from build123d import *

# Parameters (mm, degrees)
F0_W     = 3.81
F0_H     = 88.9
F1_DEPTH = 7.62


with BuildPart() as f1:
    # F0 (on Top) → F1 (new body)
    with BuildSketch(Plane.XY):
        Polygon((12.7, 0), (0, 0), (0, -21.2725), (7.62, -21.2725), (7.62, -33.9725), (0, -33.9725), (0, -46.6725), (7.62, -46.6725), (7.62, -59.3725), (0, -59.3725), (0, -72.0725), (7.62, -72.0725), (7.62, -84.7725), (0, -84.7725), (0, -97.4725), (7.62, -97.4725), (7.62, -110.1725), (0, -110.1725), (0, -131.445), (12.7, -131.445), (12.7, -123.825), (25.4, -123.825), (25.4, -131.445), (38.1, -131.445), (38.1, -123.825), (50.8, -123.825), (50.8, -131.445), (63.5, -131.445), (63.5, -123.825), (76.2, -123.825), (76.2, -131.445), (88.9, -131.445), (88.9, -110.1725), (81.28, -110.1725), (81.28, -97.4725), (88.9, -97.4725), (88.9, -84.7725), (81.28, -84.7725), (81.28, -72.0725), (88.9, -72.0725), (88.9, -59.3725), (81.28, -59.3725), (81.28, -46.6725), (88.9, -46.6725), (88.9, -33.9725), (81.28, -33.9725), (81.28, -21.2725), (88.9, -21.2725), (88.9, 0), (76.2, 0), (76.2, -7.62), (63.5, -7.62), (63.5, 0), (50.8, 0), (50.8, -7.62), (38.1, -7.62), (38.1, 0), (25.4, 0), (25.4, -7.62), (12.7, -7.62), align=None)
        with Locations((17.145, -66.04)):
            Rectangle(F0_W, F0_H, mode=Mode.SUBTRACT)
        with Locations((24.003, -66.04)):
            Rectangle(F0_W, F0_H, mode=Mode.SUBTRACT)
        with Locations((30.861, -66.04)):
            Rectangle(F0_W, F0_H, mode=Mode.SUBTRACT)
        with Locations((37.719, -66.04)):
            Rectangle(F0_W, F0_H, mode=Mode.SUBTRACT)
        with Locations((51.181, -66.04)):
            Rectangle(F0_W, F0_H, mode=Mode.SUBTRACT)
        with Locations((58.039, -66.04)):
            Rectangle(F0_W, F0_H, mode=Mode.SUBTRACT)
        with Locations((64.897, -66.04)):
            Rectangle(F0_W, F0_H, mode=Mode.SUBTRACT)
        with Locations((71.755, -66.04)):
            Rectangle(F0_W, F0_H, mode=Mode.SUBTRACT)
    extrude(amount=F1_DEPTH)


solid = f1.part
The listing builds one solid part. Answer for the finished solid, in the listing's coordinates (mm). A direction names the side the tool comes from. Give positions to 0.01 mm unless a question says otherwise; leave off trailing zeros. Answer as a JSON object with one key per item and string values.
1. Find the intervals of material crossed by L1, parallel to Y at x = 84.5, z = 0.5 (1 decimal); L2, parallel to X at y = -7, z = 1.5; L3, parallel to Y at x = 57, z = 2.75 (3 decimals), in increasing order. Write a range as [from, to].
Determined:
{"L1": "[-131.4, -110.2], [-97.5, -84.8], [-72.1, -59.4], [-46.7, -34], [-21.3, 0]", "L2": "[0, 12.7], [25.4, 38.1], [50.8, 63.5], [76.2, 88.9]", "L3": "[-131.445, -110.49], [-21.59, 0]"}
2. For faces 4 (the flat face through (0, -40, 4)), 5 (the flat face through (4, -33.972, 4)), 6 (the flat face through (50.8, -4, 4)), 7 (the flat face through (70, -123.825, 4)), 8 (the flat face through (51, -110.49, 4)), determine the directions among +Z, -Z, +X, -X, +Y, -Y from which every point of the face is accessible in a straight line to the end or side of a thin tool.
Determined:
{"face 4": "+Z, -Z, -X, +Y, -Y", "face 5": "+Z, -Z, -X", "face 6": "+Z, -Z, +Y", "face 7": "+Z, -Z, -Y", "face 8": "+Z, -Z"}
3. Flat-ended cylindrical pins translate along their axes: pin 1 Ø1 at (y, z) = (-83, 4) entering from -X; pin 2 Ø2 at (y, z) = (-53.5, 2.5) entering from +X; pin 3 Ø4 at (x, z) = (72, 3.5) entering from +Y. Find the tip coordinate at first contact, or state that the pin passes through.
Determined:
{"pin 1": "x = 7.62", "pin 2": "x = 81.28", "pin 3": "y = -7.62"}
4. For a pull along X with two mould halves and no side action, classify faces 1 (the flat face through (32.766, -67, 4)), 2 (the flat face through (0, -121, 4)), 3 (the flat face through (4, -110.172, 4)) as pulls with the +X half, pulls with the -X half, needs draft (parallel to the pull), parting line crosses it, or undercut.
Determined:
{"face 1": "undercut", "face 2": "pulls with the -X half", "face 3": "needs draft"}
5. A cutting plane is placed at A-A (y = -81). Give the number of separate pieces and of enclosed holes in the cut face, then the cut area to 3 significant figures.
Determined:
{"separate pieces": "9", "enclosed holes": "0", "area": "329 mm²"}
